Read the model definition and answer for the solid it produces. Units are mm, in the model's axes. A direction names the side the tool comes from. Coordinates: 2 decimals unless noted, no trailing zeros. Order: outer loops, then holes, each group sorted by start corner. A loop starts at its lowest first (then second) coordinate and runs counter-clockwise, first axis right, second up. Notation, with made-up numbers: M -35.5,67.5 L -8.5,67.5 A22 ccw -8.5,83.5 Z; hole C 55,86 d10. An arc over 180 degrees is marked long. Write each question's results on one line, items separated by ' | '.
```python
from build123d import *

# Parameters (mm, degrees)
EXTRUDE_1_DEPTH     = 3
EXTRUDE_2_DEPTH     = 3
EXTRUDE_3_DEPTH     = 3
SKETCH_4_R          = 1.6
CUT_EXTRUDE_1_DEPTH = 25.501881543
FILLET_1_R          = 2
SKETCH_5_W          = 0.2
SKETCH_5_H          = 2
SKETCH_5_W_2        = 2
SKETCH_5_H_2        = 0.2
EXTRUDE_4_DEPTH     = 6


with BuildPart() as part:
    # ｽｹｯﾁ1 → ﾎﾞｽ - 押し出し1 (new body)
    with BuildSketch(Plane.XY):
        with BuildLine():
            Line((-11, 8.75), (-11, -8.75))
            ThreePointArc((-11, -8.75), (0, -14.055692797), (11, -8.75))
            Line((11, -8.75), (11, 8.75))
            ThreePointArc((11, 8.75), (0, 14.055692797), (-11, 8.75))
        make_face()
    extrude(amount=EXTRUDE_1_DEPTH)

    # ｽｹｯﾁ2 → ﾎﾞｽ - 押し出し2 (add)
    with BuildSketch(Plane.XY.offset(3)):
        with BuildLine():
            Line((-11, 8.75), (-11, 17.75))
            Line((-11, 17.75), (0, 21.055692797))
            Line((0, 21.055692797), (0, 14.055692797))
            ThreePointArc((0, 14.055692797), (6.106356853, 12.65997259), (11, 8.75))
            Line((11, 8.75), (11, -8.75))
            Line((11, -8.75), (11, -17.75))
            Line((11, -17.75), (0, -21.055692797))
            Line((0, -21.055692797), (0, -14.055692797))
            ThreePointArc((0, -14.055692797), (-6.106356853, -12.65997259), (-11, -8.75))
            Line((-11, -8.75), (-11, 8.75))
        make_face()
    extrude(amount=EXTRUDE_2_DEPTH)

    # ｽｹｯﾁ3 → ﾎﾞｽ - 押し出し3 (add)
    with BuildSketch(Plane.XY.offset(6)):
        with BuildLine():
            Line((-11, 8.75), (-11, -8.75))
            ThreePointArc((-11, -8.75), (0, -14.055692797), (11, -8.75))
            Line((11, -8.75), (11, 8.75))
            ThreePointArc((11, 8.75), (0, 14.055692797), (-11, 8.75))
        make_face()
    extrude(amount=EXTRUDE_3_DEPTH)

    # ｽｹｯﾁ4 → ｶｯﾄ - 押し出し1 (cut, through all)
    with BuildSketch(Plane.XY.offset(6)):
        with Locations((-7, 15.452070108)):
            Circle(SKETCH_4_R)
        with Locations((7, -15.452070108)):
            Circle(SKETCH_4_R)
    extrude(amount=-CUT_EXTRUDE_1_DEPTH, mode=Mode.SUBTRACT)

    # ﾌｨﾚｯﾄ1
    fillet_1_edges = [part.edges().sort_by_distance(p)[0] for p in [
        (0, -21.055692797, 4.5),
        (11, -17.75, 4.5),
        (0, 21.055692797, 4.5),
        (-11, 17.75, 4.5),
    ]]
    fillet(fillet_1_edges, radius=FILLET_1_R)

    # ｽｹｯﾁ5 → ﾎﾞｽ - 押し出し4 (add)
    with BuildSketch(Plane.XY.offset(9)):
        Polygon((3.947100797, 9.79045687), (3.181733933, 7.942697805), (3.366509839, 7.866161118), (4.131876704, 9.713920183), align=None)
        with Locations((0, 9.555692797)):
            Rectangle(SKETCH_5_W, SKETCH_5_H)
        Polygon((7.393291279, 7.534712635), (5.979077716, 6.120499073), (6.120499073, 5.979077716), (7.534712635, 7.393291279), align=None)
        Polygon((7.534712635, -7.393291279), (6.120499073, -5.979077716), (5.979077716, -6.120499073), (7.393291279, -7.534712635), align=None)
        Polygon((4.131876704, -9.713920183), (3.366509839, -7.866161118), (3.181733933, -7.942697805), (3.947100797, -9.79045687), align=None)
        with Locations((0, -9.555692797)):
            Rectangle(SKETCH_5_W, SKETCH_5_H)
        Polygon((-3.947100797, -9.79045687), (-3.181733933, -7.942697805), (-3.366509839, -7.866161118), (-4.131876704, -9.713920183), align=None)
        Polygon((-7.393291279, -7.534712635), (-5.979077716, -6.120499073), (-6.120499073, -5.979077716), (-7.534712635, -7.393291279), align=None)
        Polygon((-7.534712635, 7.393291279), (-6.120499073, 5.979077716), (-5.979077716, 6.120499073), (-7.393291279, 7.534712635), align=None)
        Polygon((-4.131876704, 9.713920183), (-3.366509839, 7.866161118), (-3.181733933, 7.942697805), (-3.947100797, 9.79045687), align=None)
        with Locations((-6.5, 0)):
            Rectangle(SKETCH_5_W_2, SKETCH_5_H_2)
        with Locations((6.5, 0)):
            Rectangle(SKETCH_5_W_2, SKETCH_5_H_2)
    extrude(amount=EXTRUDE_4_DEPTH)


solid = part.part
```
(1) The part is cut by section A-A, the plane y = -14.5. Write down the section's boundary in (x, z).
Conclusion:
outline: M 0,3 L 5.71,3 L 5.71,6 L 0,6 Z; M 8.29,3 L 11,3 L 11,6 L 8.29,6 Z
(2) The part is cut by section B-B, the plane x = -7. Write down the section's boundary in (y, z), then the cut area to 3 significant figures.
Conclusion:
outline: M -12.19,0 L 12.19,0 L 12.19,3 L 13.85,3 L 13.85,6 L 12.19,6 L 12.19,9 L 7.14,9 L 7.14,15 L 6.86,15 L 6.86,9 L 0.1,9 L 0.1,15 L -0.1,15 L -0.1,9 L -6.86,9 L -6.86,15 L -7.14,15 L -7.14,9 L -12.19,9 Z; M 17.05,3 L 18.95,3 L 18.95,6 L 17.05,6 Z | area: 235 mm²
(3) The part is cut by section C-C, the plane z = 9.75. Count the separate pieces of the cut face and the enclosed holes in it, then the cut area to 3 significant figures.
Conclusion:
separate pieces: 12 | enclosed holes: 0 | area: 4.80 mm²
(4) The part is cut by section D-D, the plane x = 1.75. Write down the section's boundary in (y, z), then the cut area to 3 significant figures.
Conclusion:
outline: M -20.35,3 L -13.95,3 L -13.95,0 L 13.95,0 L 13.95,9 L -13.95,9 L -13.95,6 L -20.35,6 Z | area: 270 mm²
(5) For faces 1 (the flat face through (-7, -0.1, 12)), 2 (the flat face through (0.1, -10, 12)), 3 (the flat face through (6.82, 6.68, 11.96)), 4 (the flat face through (-6.84, 6.7, 11.96)), determine the directions among +Z, -Z, +X, -X, +Y, -Y from which every point of the face is accessible in a straight line to the end or side of a thin tool.
Conclusion:
face 1: +Z, +X, -X | face 2: +Z, +Y, -Y | face 3: +Z, +X | face 4: +Z, -X
(6) The mould has two halves that part along X. Classify faces 5 (the flat face through (3.744, 8.777, 11.958)), 6 (the flat face through (-6.68, 6.82, 11.96)), 7 (the flat face through (-7, 0.1, 12)): pulls with the +X half, pulls with the -X half, needs draft (parallel to the pull), parting line crosses it, or undercut.
Conclusion:
face 5: pulls with the +X half | face 6: undercut | face 7: needs draft
(7) Given pin 1 (5.5 mm diameter, centred on x = 8, y = -13.5, fed in from +Z); pin 2 (2 mm diameter, centred on y = 13.5, z = 4.5, fed in from +X); pin 3 (1.6 mm diameter, centred on x = 6, z = 13.5, fed in from -Y), each flat-ended and moving along its own axis, determine where each tip first touches the part or whether it passes through.
Conclusion:
pin 1: z = 9 | pin 2: x = 6.43 | pin 3: y = -6.94
(8) Straight lines are drawn through the part: line 1 (Y direction, x = 7, z = 5.25); line 2 (Y direction, x = -7, z = 3.95); line 3 (Z direction, x = -4.25, y = 9.5). For each, find the intervals that lie inside material, in ascending order.
Conclusion:
line 1: -18.95 to -17.05, -13.85 to 12.19 | line 2: -12.19 to 13.85, 17.05 to 18.95 | line 3: 0 to 9
